Source: three-view drawing plus pictorial views. Frame: mm from the lowest corner of the part. A direction names the side the tool comes from. Give positions to 0.01 mm unless a question says otherwise; leave off trailing zeros. Order: outer loops, then holes, each group sorted by start corner. A loop starts at its lowest first (then second) coordinate and runs counter-clockwise, first axis right, second up. Notation, with made-up numbers: (14.5, 50) - (36.5, 50) arc R24 cw to (36.5, 67) - close; hole circle Ø4 at (55, 7). An arc over 180 degrees is marked (long way). Answer in a Markdown table with one row per item. Add a question column.
1. Mould query, pull axis Y, two halves, no side actions, for the marked faces 1, 2, 3 and 4. Classes: released by +Y, released by -Y, zero draft, split by the parting line, or undercut.
2. Access query for the marked faces 5 and 6. Directions: +Z, -Z, +X, -X, +Y, -Y. A direction counts if a zero-diameter tool reaches every point of the face in a straight line with its end or side. Return the directions, or none.
3. Section query B-B on y = 41.5. Return loops of the section in (x, z).
4. Contact query for flat-ended pins moving along their axis: pin 1 (5 mm diameter, centred on x = 16, y = 76.5, fed in from -Z); pin 2 (5 mm diameter, centred on x = 40, z = 19.5, fed in from -Y). Output: stop coordinate, or through.
5. Section query C-C on x = 55.5. Return loops of the section in (y, z), and give its area (3 significant figures).
6. Section query A-A on z = 11.5. Return loops of the section in (x, y), and give its area (3 significant figures).
7. Ray query, line 1 (Y direction, x = 81, z = 11.75); line 2 (X direction, y = 68, z = 11.5); line 3 (Z direction, x = 50, y = 49). Return the intervals inside material, ascending. Write a range as [from, to].
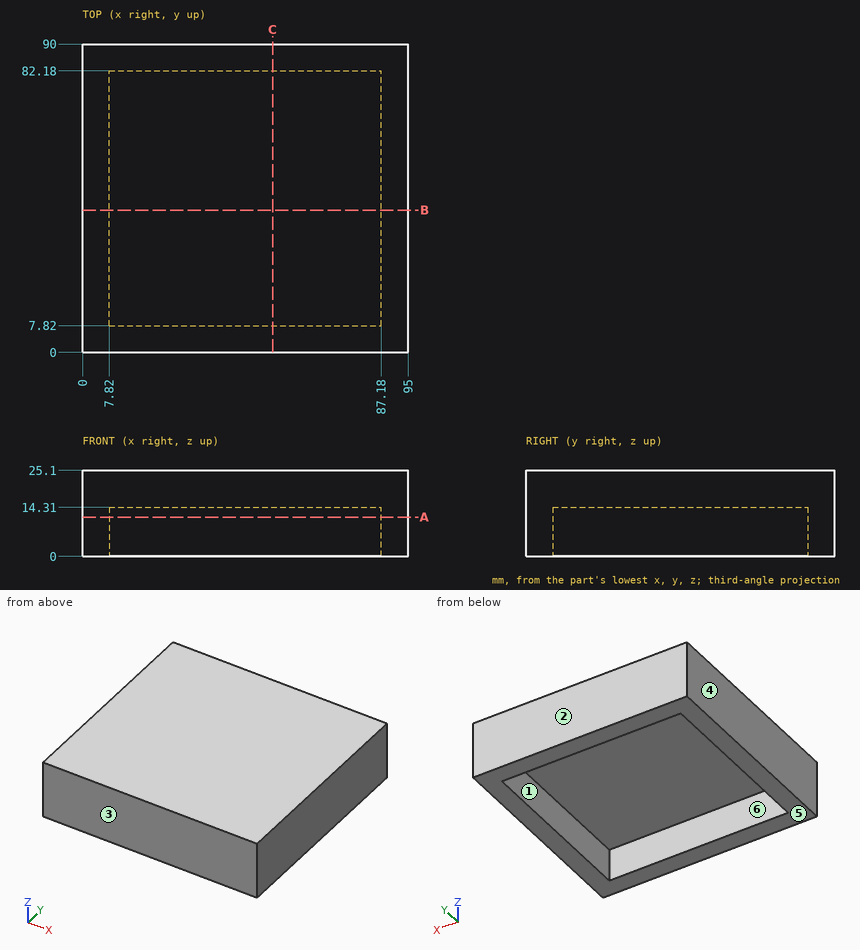
Answer:
| question | item | result |
|---|---|---|
| 1 | face 1 | undercut |
| 1 | face 2 | released by +Y |
| 1 | face 3 | released by -Y |
| 1 | face 4 | zero draft |
| 2 | face 5 | -Z, +X, -X, +Y, -Y |
| 2 | face 6 | -Z |
| 3 | outline | (0, 0) - (7.82, 0) - (7.82, 14.31) - (87.18, 14.31) - (87.18, 0) - (95, 0) - (95, 25.1) - (0, 25.1) - close |
| 4 | pin 1 | stops at z = 14.31 |
| 4 | pin 2 | stops at y = 0 |
| 5 | outline | (0, 0) - (7.82, 0) - (7.82, 14.31) - (82.18, 14.31) - (82.18, 0) - (90, 0) - (90, 25.1) - (0, 25.1) - close |
| 5 | area | 1,190 mm² |
| 6 | outline | (0, 0) - (95, 0) - (95, 90) - (0, 90) - close; hole (7.82, 7.82) - (87.18, 7.82) - (87.18, 82.18) - (7.82, 82.18) - close |
| 6 | area | 2,650 mm² |
| 7 | line 1 | y = [0, 7.82], [82.18, 90] |
| 7 | line 2 | x = [0, 7.82], [87.18, 95] |
| 7 | line 3 | z = [14.31, 25.1] |
